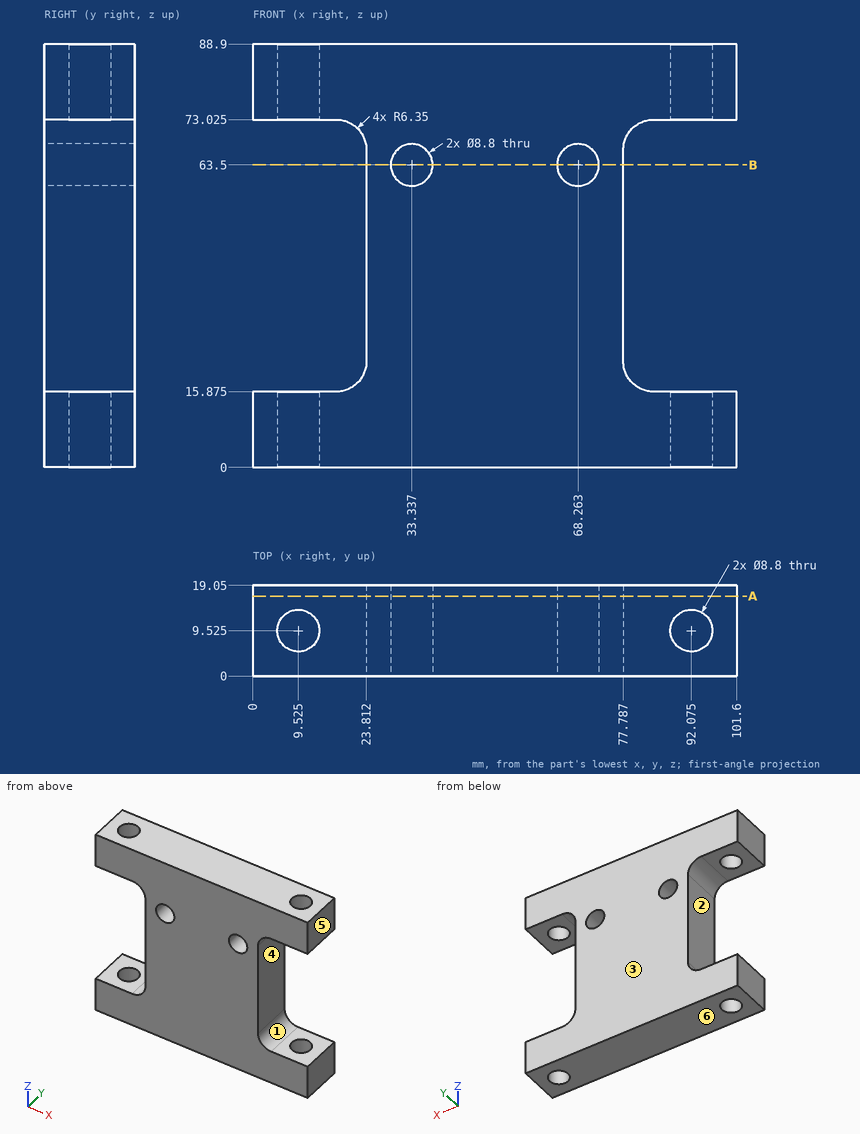
Could you check a few things on this drawing? It's one solid part, dimensions in mm from its lowest x, y, z. A direction names the side the tool comes from. Round coordinates to 2 decimals unless told otherwise and drop trailing zeros. Order: outer loops, then holes, each group sorted by start corner. A loop starts at its lowest first (then second) coordinate and runs counter-clockwise, first axis right, second up. Notation, with made-up numbers: M 16,71 L 41,71 A26 ccw 41,90 Z; hole C 10,55.5 d8. An arc over 180 degrees is marked long. One line per question, with ' | ' between items.
1) Imagine slicing it at A-A, the plane y = 16.75. Count the separate pieces of the cut face and the enclosed holes in it, plus the area to 3 significant figures.
Checked values:
separate pieces: 1 | enclosed holes: 2 | area: 6,220 mm²
2) I'm going to push flat-ended pins straight in: pin 1 Ø5.5 at (y, z) = (13, 39.5) entering from -X; pin 2 Ø10 at (x, y) = (9.525, 9.525) entering from +Z; pin 3 Ø1 at (y, z) = (12, 23.5) entering from +X. Where does each tip first touch, or does it pass through?
Checked values:
pin 1: stops at x = 23.81 | pin 2: stops at z = 88.9 | pin 3: stops at x = 77.79
3) Imagine slicing it at B-B, the plane z = 63.5. Write out the boundary of the cut face in (x, y).
Checked values:
outline: M 23.81,0 L 28.94,0 L 28.94,19.05 L 23.81,19.05 Z; M 37.74,0 L 63.86,0 L 63.86,19.05 L 37.74,19.05 Z; M 72.66,0 L 77.79,0 L 77.79,19.05 L 72.66,19.05 Z
4) On a 3-axis mill with a long thin cutter (end or side, diameter ignored), from which of +Z, -Z, +X, -X, +Y, -Y can I reach the whole of each face in a straight line? I mean the marked faces 1, 2 and 3. Say none if no direction works.
Checked values:
face 1: +X, +Y, -Y | face 2: -X, +Y, -Y | face 3: +Z, -Z, +X, -X, +Y
5) We'd pull the mould along Z, two halves only. Please class the marked faces 4, 5 and 6: released by +Z, released by -Z, zero draft, split by the parting line, or undercut.
Checked values:
face 4: undercut | face 5: zero draft | face 6: released by -Z
6) I need wall thicknesses on line 1 (X direction, y = 4.25, z = 63.5); line 2 (Z direction, x = 84, y = 13.75); line 3 (X direction, y = 14, z = 66.5) (1 decimal). Which ranges of each line are inside material? Lowest first, please.
Checked values:
line 1: x = 23.81 to 28.94, 37.74 to 63.86, 72.66 to 77.79 | line 2: z = 0 to 15.88, 73.02 to 88.9 | line 3: x = 23.8 to 30.1, 36.6 to 65, 71.5 to 77.8
